Model file for the job. Use its own axes, mm. A direction names the side the tool comes from. Give positions to 0.01 mm unless a question says otherwise; leave off trailing zeros. Write each loop counter-clockwise with the first axis right and the second up, starting at its lowest first coordinate (ties: lowest second). Pieces come first, ordered by that corner, then holes. Notation, with made-up numbers: (23, 84.5) - (70, 84.5) arc R12 ccw to (70, 88.5) - close; hole circle Ø10 at (35.25, 2). An arc over 180 degrees is marked (long way). One line per item, written item: value. Start each with the question number.
(1) Probe L1, parallel to Z at x = -0.4, y = 1.3; L2, parallel to Y at x = -1.3, z = -3.25; L3, parallel to X at y = 0.8, z = -4. List the from-to ranges inside material, lowest first.
(2) Cut at C-C, the plane z = 3.25. List the corners of the cut face in (x, y).
(3) Mould opens along Y. For faces 1 (the face through (-3, 0, 0)), 2 (the face through (0, -2, -6)), 3 (the face through (0, -1.5, -4)) say: pulls with the +Y half, pulls with the -Y half, needs draft (parallel to the pull), parting line crosses it, or undercut.
(4) 3-axis set-ups, long thin cutter, end or side, ignore diameter. For faces 4 (the face through (-1.427, -0.761, -4.028)), 5 (the face through (0, 0, 6)): which of +Z, -Z, +X, -X, +Y, -Y reach the whole face in a straight line?
(5) Cut at A-A, the plane z = -4.5. List the corners of the cut face in (x, y), and give its area (3 significant figures).
(6) Drop flat-ended pins along their axis: P1, Ø1.5, axis at x = -2, z = 2.5, coming from the -Y side; P2, Ø1, axis at y = 1.5, z = -4.5, coming from the -X side. Give the stop position or say it passes through.
(7) Cut at B-B, the plane x = 0. List the corners of the cut face in (y, z).
Autodesk Inventor part; units mm, degrees
ref_plane "YZ Plane" through (0, 0, 0) normal (1, 0, 0) x (0, 1, 0)
ref_plane "XZ Plane" through (0, 0, 0) normal (0, 1, 0) x (-1, 0, 0)
ref_plane "XY Plane" through (0, 0, 0) normal (0, 0, 1) x (1, 0, 0)
sketch "Sketch1" plane through (0, 0, 0) normal (0, 0, 1) x (1, 0, 0)
  circle A0 centre (0, 0) radius 3
  dimension "d0" = 6
extrude "Extrusion1" add sketch "Sketch1" along normal mid plane 12
chamfer "Chamfer1" distance 0.5 angle 45 2 edges at (-3, 0, 6) (-3, 0, -6)
sketch "Sketch2" plane through (0, 0, -6) normal (0, 0, -1) x (-1, 0, 0)
  circle A0 centre (0, 0) radius 2.5
  line L0 (-1.866, 0) -> (-1, -1.5)
  line L1 (-1, 1.5) -> (-1.866, 0)
  line L2 (1, 1.5) -> (-1, 1.5)
  line L3 (1.866, 0) -> (1, 1.5)
  line L4 (1, -1.5) -> (1.866, 0)
  line L5 (-1, -1.5) -> (1, -1.5)
  circle A1 centre (0, 0) radius 1.616 construction
  dimension "d5" = 3.2321
  dimension "d10" = 1.5
  dimension "d11" = 120
  dimension "d13" = 120
  dimension "d16" = 3
extrude "Extrusion2" cut sketch "Sketch2" against normal blind 4 contours L1 L2 L3 L4 L5 L0
thread "Thread1"
properties part number "6mm SHCS"
Answers follow:
1. L1: z = -2 to 6
1. L2: y = -2.7 to -0.98, 0.98 to 2.7
1. L3: x = -2.89 to -1.4, 1.4 to 2.89
2. outline: circle Ø6 at (0, 0)
3. face 1: parting line crosses it
3. face 2: needs draft
3. face 3: undercut
4. face 4: -Z
4. face 5: +Z, +X, -X, +Y, -Y
5. outline: circle Ø6 at (0, 0); hole (-1.87, 0) - (-1, -1.5) - (1, -1.5) - (1.87, 0) - (1, 1.5) - (-1, 1.5) - close
5. area: 19.7 mm²
6. P1: stops at y = -2.73
6. P2: stops at x = -2.83
7. outline: (-3, -5.5) - (-2.5, -6) - (-1.5, -6) - (-1.5, -2) - (1.5, -2) - (1.5, -6) - (2.5, -6) - (3, -5.5) - (3, 5.5) - (2.5, 6) - (-2.5, 6) - (-3, 5.5) - close
